Build history of the part. All positions in model axes, mm. Face numbers are marked on the shaded views. Round coordinates to 2 decimals unless told otherwise and drop trailing zeros. Write each loop counter-clockwise with the first axis right and the second up, starting at its lowest first coordinate (ties: lowest second). Pieces come first, ordered by that corner, then holes.
Item 1: Band-saw the part on A-A, the plane z = 0. Write the cut outline in (x, y), then the cut area to 3 significant figures.
Item 2: Band-saw the part on B-B, the plane z = 2.5. Write the cut outline in (x, y), then the cut area to 3 significant figures.
Item 3: Drop flat-ended pins along their axis: pin 1 Ø5 at (x, y) = (26.5, -1.5) entering from -Z; pin 2 Ø3 at (y, z) = (-11, 1.5) entering from -X; pin 3 Ø1.5 at (x, z) = (12.5, -2.5) entering from +Y. Give the stop position or say it passes through.
Item 4: Mould opens along X. For the marked faces 1, 2, 3 and 4 say: +X half, -X half, draft (parallel to the pull), parting line (faces both ways), or undercut.
Item 5: Wall check: probe 1 along Z at (x, y) = (9, 0); probe 2 along X at (y, z) = (-15.5, 1); probe 3 along X at (y, z) = (-13.25, 1.25). Give the ranges that are in metal, low to high.
Item 6: Band-saw the part on C-C, the plane x = 24.5. Write the cut outline in (y, z).
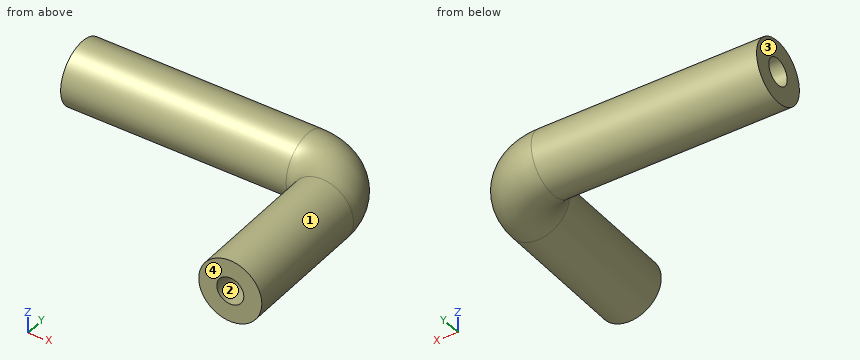
Autodesk Inventor part; units mm, degrees
ref_plane "YZ Plane" through (0, 0, 0) normal (1, 0, 0) x (0, 1, 0)
ref_plane "XZ Plane" through (0, 0, 0) normal (0, 1, 0) x (-1, 0, 0)
ref_plane "XY Plane" through (0, 0, 0) normal (0, 0, 1) x (1, 0, 0)
sketch "Sketch2" plane through (0, 0, 0) normal (1, 0, 0) x (0, 1, 0)
  circle A0 centre (0, 0) radius 1.5
  circle A1 centre (0, 0) radius 3.5
  dimension "d8" = 3
  dimension "d9" = 2
sketch3d "3D Sketch1"
  line L0 (0, 0, 0) -> (25, 0, 0)
  arc A0 (25, 0, 0) -> (30, -5, 0) centre (25, -5, 0) ccw
  line L1 (30, -5, 0) -> (30, -20, 0)
  dimension "d3" = 30
  dimension "d4" = 20
  dimension "d6" = 5
sweep "Sweep1" add profiles "Sketch2" path "3D Sketch1"
properties part number "Pipe3"
Results:
1. outline: (0, -3.5) - (25, -3.5) arc R1.5 cw to (26.5, -5) - (26.5, -20) - (28.5, -20) - (28.5, -5) arc R3.5 ccw to (25, -1.5) - (0, -1.5) - close; (0, 1.5) - (25, 1.5) arc R6.5 cw to (31.5, -5) - (31.5, -20) - (33.5, -20) - (33.5, -5) arc R8.5 ccw to (25, 3.5) - (0, 3.5) - close
1. area: 191 mm2
2. outline: (0, -2.45) - (25, -2.45) arc R2.55 cw to (27.55, -5) - (27.55, -20) - (32.45, -20) - (32.45, -5) arc R7.45 ccw to (25, 2.45) - (0, 2.45) - close
2. area: 234 mm2
3. pin 1: stops at z = -3.5
3. pin 2: stops at x = 26.5
3. pin 3: stops at y = 3.03
4. face 1: parting line
4. face 2: undercut
4. face 3: -X half
4. face 4: draft
5. probe 1: z = -3.5 to -1.5, 1.5 to 3.5
5. probe 2: x = 26.65 to 28.88, 31.12 to 33.35
5. probe 3: x = 26.73 to 29.17, 30.83 to 33.27
6. outline: circle Ø7 at (0, 0); hole circle Ø3 at (0, 0)
